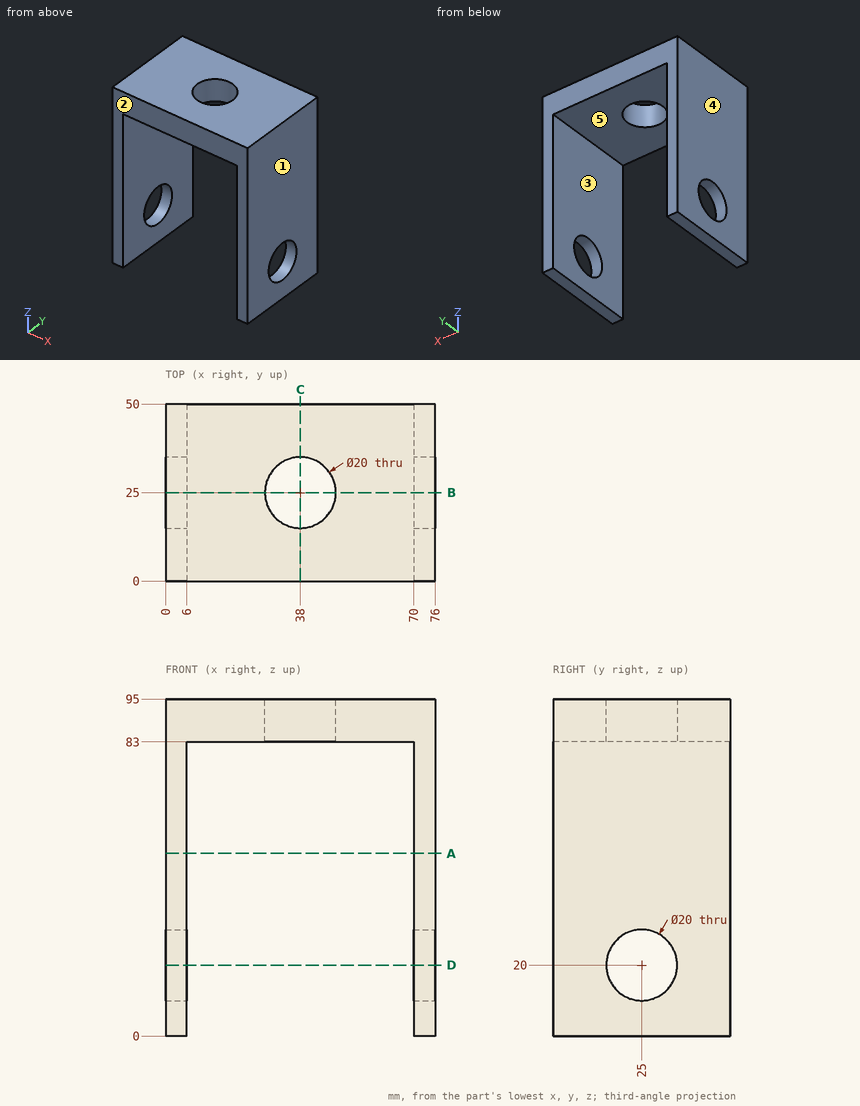
The figure shows three views and two pictorial views of one solid part (mm, origin at its lowest corner). Answer the questions. A direction names the side the tool comes from. Coordinates: 2 decimals unless noted, no trailing zeros. Loops run counter-clockwise (first coordinate to the right, second up) from the corner with the lowest first, then second, coordinate; pieces in that order, holes last. Notation, with made-up numbers: M 79.25,65.5 L 127.25,65.5 A29 ccw 127.25,89.5 Z; hole C -18,23.5 d10. An arc over 180 degrees is marked long. Use CSV: the item, a comma, the result in double quotes. Start each with the question number.
(1) Find section D-D, the plane z = 20. Give the vertices of the cut face in (x, y), then the cut area to 3 significant figures.
(2) Find section B-B, the plane y = 25. Give the vertices of the cut face in (x, z).
(3) Given pin 1 Ø23 at (x, y) = (38, 25) entering from -Z; pin 2 Ø2 at (y, z) = (8.5, 79.5) entering from -X, each flat-ended and moving along its own axis, determine where each tip first touches the part or whether it passes through.
(4) Find section A-A, the plane z = 51.5. Give the vertices of the cut face in (x, y).
(5) For a pull along X with two mould halves and no side action, classify the marked faces 1, 2 and 3 as +X half, -X half, draft (parallel to the pull), parting line (faces both ways), or undercut.
(6) For the marked faces 4 and 5, determine the directions among +Z, -Z, +X, -X, +Y, -Y from which every point of the face is accessible in a straight line to the end or side of a thin tool.
(7) Consider line 1 (X direction, y = 18.5, z = 40); line 2 (Z direction, x = 2.5, y = 25); line 3 (Y direction, x = 38, z = 87). Determine where each line is inside the solid, lowest interval first.
(8) Find section C-C, the plane x = 38. Give the vertices of the cut face in (y, z).
Recorded:
1,outline,"M 0,0 L 6,0 L 6,15 L 0,15 Z; M 0,35 L 6,35 L 6,50 L 0,50 Z; M 70,0 L 76,0 L 76,15 L 70,15 Z; M 70,35 L 76,35 L 76,50 L 70,50 Z"
1,area,"360 mm^2"
2,outline,"M 0,0 L 6,0 L 6,10 L 0,10 Z; M 0,30 L 6,30 L 6,83 L 28,83 L 28,95 L 0,95 Z; M 48,83 L 70,83 L 70,30 L 76,30 L 76,95 L 48,95 Z; M 70,0 L 76,0 L 76,10 L 70,10 Z"
3,pin 1,"stops at z = 83"
3,pin 2,"stops at x = 0"
4,outline,"M 0,0 L 6,0 L 6,50 L 0,50 Z; M 70,0 L 76,0 L 76,50 L 70,50 Z"
5,face 1,"+X half"
5,face 2,"draft"
5,face 3,"undercut"
6,face 4,"+Z, -Z, -X, +Y, -Y"
6,face 5,"-Z, +Y, -Y"
7,line 1,"x = 0 to 6, 70 to 76"
7,line 2,"z = 0 to 10, 30 to 95"
7,line 3,"y = 0 to 15, 35 to 50"
8,outline,"M 0,83 L 15,83 L 15,95 L 0,95 Z; M 35,83 L 50,83 L 50,95 L 35,95 Z"
